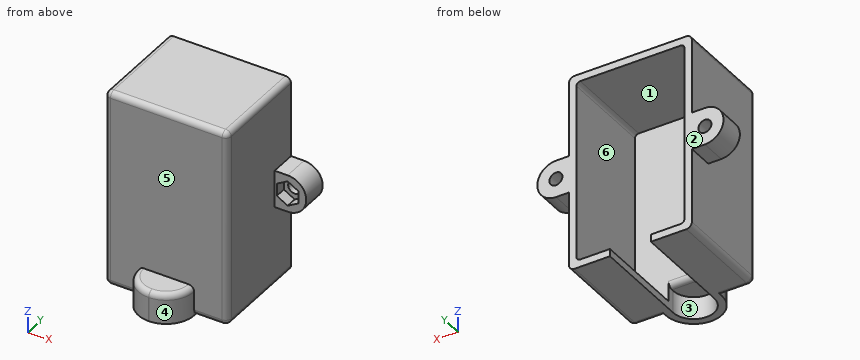
from build123d import *

# Parameters (mm, degrees)
SKETCH_R        = 1.75
PAD_DEPTH       = 27
SKETCH001_W     = 29
SKETCH001_H     = 49
POCKET_DEPTH    = 25
SKETCH002_W     = 9
SKETCH002_H     = 10
POCKET001_DEPTH = 20
POCKET002_DEPTH = 3
PAD001_DEPTH    = 8
POCKET003_DEPTH = 6
FILLET_R        = 1.5
FILLET001_R     = 1.5
FILLET002_R     = 1.5
FILLET003_R     = 1


with BuildPart() as part:
    # Sketch → Pad (new body)
    with BuildSketch(Plane.XZ):
        with BuildLine():
            Line((-16.5, 26.5), (16.5, 26.5))
            Line((16.5, 26.5), (16.5, 5))
            Line((16.5, 5), (20, 5))
            ThreePointArc((20, -5), (25, 0), (20, 5))
            Line((20, -5), (16.5, -5))
            Line((16.5, -5), (16.5, -26.5))
            Line((16.5, -26.5), (-16.5, -26.5))
            Line((-16.5, -26.5), (-16.5, -5))
            Line((-20, -5), (-16.5, -5))
            ThreePointArc((-20, 5), (-25, 0), (-20, -5))
            Line((-16.5, 5), (-20, 5))
            Line((-16.5, 5), (-16.5, 26.5))
        make_face()
        with Locations((-20, 0)):
            Circle(SKETCH_R, mode=Mode.SUBTRACT)
        with Locations((20, 0)):
            Circle(SKETCH_R, mode=Mode.SUBTRACT)
    extrude(amount=PAD_DEPTH)

    # Sketch001 (on Face15 of Pad) → Pocket (cut)
    with BuildSketch(Plane(origin=(0, 0, 0), x_dir=(1, 0, 0), z_dir=(0, 1, 0))):
        Rectangle(SKETCH001_W, SKETCH001_H)
    extrude(amount=-POCKET_DEPTH, mode=Mode.SUBTRACT)

    # Sketch002 (on Face5 of Pocket) → Pocket001 (cut)
    with BuildSketch(Plane.XZ.offset(27)):
        with Locations((-21, 0)):
            Rectangle(SKETCH002_W, SKETCH002_H)
        with Locations((21, 0)):
            Rectangle(SKETCH002_W, SKETCH002_H)
    extrude(amount=-POCKET001_DEPTH, mode=Mode.SUBTRACT)

    # Sketch003 (on Face8 of Pocket001) → Pocket002 (cut)
    with BuildSketch(Plane.XZ.offset(7)):
        Polygon((-17.1, 1.674316), (-20, 3.348632), (-22.9, 1.674316), (-22.9, -1.674316), (-20, -3.348632), (-17.1, -1.674316), align=None)
        Polygon((22.9, 1.674316), (20, 3.348632), (17.1, 1.674316), (17.1, -1.674316), (20, -3.348632), (22.9, -1.674316), align=None)
    extrude(amount=-POCKET002_DEPTH, mode=Mode.SUBTRACT)

    # Sketch004 (on Face14 of Pocket002) → Pad001 (join)
    with BuildSketch(Plane(origin=(0, 0, -26.5), x_dir=(1, 0, 0), z_dir=(0, 0, -1))):
        with BuildLine():
            Line((-7.5, 27), (7.5, 27))
            Line((7.5, 27), (7.5, 27.01))
            ThreePointArc((7.5, 27.01), (5.30623, 32.30623), (0.01, 34.5))
            Line((0.01, 34.5), (-0.01, 34.5))
            ThreePointArc((-0.01, 34.5), (-5.30623, 32.30623), (-7.5, 27.01))
            Line((-7.5, 27.01), (-7.5, 27))
        make_face()
    extrude(amount=-PAD001_DEPTH)

    # Sketch005 (on Face14 of Pad001) → Pocket003 (cut)
    with BuildSketch(Plane(origin=(0, 0, -26.5), x_dir=(1, 0, 0), z_dir=(0, 0, -1))):
        with BuildLine():
            Line((-5.5, 0), (5.5, 0))
            Line((5.5, 0), (5.5, 27))
            ThreePointArc((5.5, 27), (0, 32.5), (-5.5, 27))
            Line((-5.5, 27), (-5.5, 0))
        make_face()
    extrude(amount=-POCKET003_DEPTH, mode=Mode.SUBTRACT)

    # Fillet
    fillet_edges = [part.edges().sort_by_distance(p)[0] for p in [
        (16.5, -13.5, 26.5),
        (-16.5, -13.5, 26.5),
        (-16.5, -13.5, -26.5),
        (16.5, -13.5, -26.5),
    ]]
    fillet(fillet_edges, radius=FILLET_R)

    # Fillet001
    fillet001_edges = [part.edges().sort_by_distance(p)[0] for p in [
        (-16.5, -27, -15),
    ]]
    fillet(fillet001_edges, radius=FILLET001_R)

    # Fillet002
    fillet002_edges = [part.edges().sort_by_distance(p)[0] for p in [
        (0, -25, -20.5),
        (5.30623, -32.30623, -18.5),
    ]]
    fillet(fillet002_edges, radius=FILLET002_R)

    # Fillet003
    fillet003_edges = [part.edges().sort_by_distance(p)[0] for p in [
        (14.5, -12.5, -24.5),
        (-14.5, -12.5, -24.5),
        (-14.5, -12.5, 24.5),
        (14.5, -12.5, 24.5),
    ]]
    fillet(fillet003_edges, radius=FILLET003_R)


solid = part.part
Here's how the part is built. I have some questions about the finished solid (model axes, mm). Face numbers are marked on the shaded views. A direction names the side the tool comes from. Coordinates: 2 decimals unless noted, no trailing zeros. Loops run counter-clockwise (first coordinate to the right, second up) from the corner with the lowest first, then second, coordinate; pieces in that order, holes last. Notation, with made-up numbers: (-12.5, 16) -> (1.5, 16) arc R24 cw to (1.5, 55) -> close; hole circle Ø6 at (-30, -3.75). An arc over 180 degrees is marked (long way). Use one line per item in the form item = value. Start each with the question number.
(1) Please list where these lines run through material, in increasing order: line 1 along X through (y, z) = (-1, 0); line 2 along X through (y, z) = (-10, -8); line 3 along Z through (x, y) = (11, -19.5).
(2) If we section it at C-C (z = -7.5): Please give me the cut outline in (x, y), then the cut area to 3 significant figures.
(3) If we section it at B-B (y = -21): Please give me the cut outline in (x, z), then the cut area to 3 significant figures.
(4) We'd pull the mould along X, two halves only. Please class the marked faces 4, 5 and 6: pulls with the +X half, pulls with the -X half, needs draft (parallel to the pull), parting line crosses it, or undercut.
(5) If we section it at A-A (z = 0): Give the number of separate pieces and of enclosed holes in the cut face, then the cut area to 3 significant figures.
(6) On a 3-axis mill with a long thin cutter (end or side, diameter ignored), from which of +Z, -Z, +X, -X, +Y, -Y can I reach the whole of each face in a straight line? I mean the marked faces 1, 2 and 3. Say none if no direction works.
(7) Will these pins go through, and if not, where does the flat tip stop? pin 1 (23 mm diameter, centred on x = 2.5, z = -0.5, fed in from +Y); pin 2 (15 mm diameter, centred on x = -0.5, z = -0.5, fed in from -Y); pin 3 (7.5 mm diameter, centred on y = -14.5, z = -5.5, fed in from +X).
Verdict:
q1.line_1 = -25 to -21.75, -18.25 to -14.5, 14.5 to 18.25, 21.75 to 25
q1.line_2 = -16.5 to -14.5, 14.5 to 16.5
q1.line_3 = -26.5 to -24.5, 24.5 to 26.5
q2.outline = (-16.5, -25.5) arc R1.5 ccw to (-15, -27) -> (15, -27) arc R1.5 ccw to (16.5, -25.5) -> (16.5, 0) -> (14.5, 0) -> (14.5, -25) -> (-14.5, -25) -> (-14.5, 0) -> (-16.5, 0) -> close
q2.area = 165 mm²
q3.outline = (-16.5, -25) arc R1.5 ccw to (-15, -26.5) -> (-5.5, -26.5) -> (-5.5, -24.5) -> (-13.5, -24.5) arc R1 cw to (-14.5, -23.5) -> (-14.5, 23.5) arc R1 cw to (-13.5, 24.5) -> (13.5, 24.5) arc R1 cw to (14.5, 23.5) -> (14.5, -23.5) arc R1 cw to (13.5, -24.5) -> (5.5, -24.5) -> (5.5, -26.5) -> (15, -26.5) arc R1.5 ccw to (16.5, -25) -> (16.5, 25) arc R1.5 ccw to (15, 26.5) -> (-15, 26.5) arc R1.5 ccw to (-16.5, 25) -> close
q3.area = 305 mm²
q4.face_4 = pulls with the +X half
q4.face_5 = needs draft
q4.face_6 = undercut
q5.separate_pieces = 3
q5.enclosed_holes = 0
q5.area = 221 mm²
q6.face_1 = +Y
q6.face_2 = +Z, -Z, +X, -X, +Y
q6.face_3 = -Z, +Y
q7.pin_1 = -25
q7.pin_2 = -27
q7.pin_3 = 16.5
